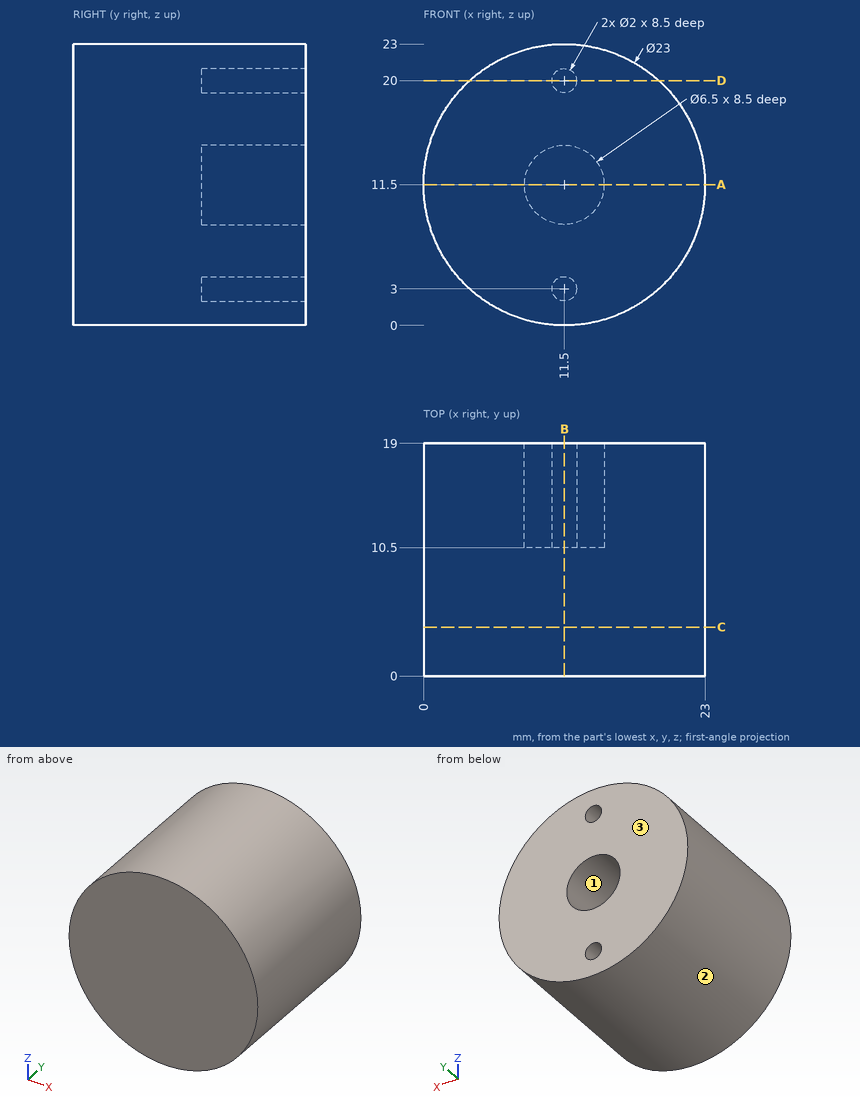
Check sheet for the drawn part. Datum: minimum x, y, z corner. Units: mm. Round coordinates to 2 decimals unless told otherwise and drop trailing zeros. Order: outer loops, then holes, each group sorted by start corner. A loop starts at its lowest first (then second) coordinate and runs counter-clockwise, first axis right, second up. Notation, with made-up numbers: M 12.25,28.5 L 41.25,28.5 A10 ccw 41.25,42.5 Z; hole C 74,17 d5. An arc over 180 degrees is marked long. Write each question's results on one line, items separated by ' | '. Start each with the question number.
1. Go/stop test with flat-tipped pins: P1, Ø0.6, axis at x = 11.5, z = 3, coming from the +Y side; P2, Ø2, axis at x = 13.5, y = 14, coming from the +Z side; P3, Ø1.2, axis at x = 11.5, z = 20, coming from the -Y side; P4, Ø5, axis at y = 5.5, z = 18, coming from the -X side. Record where each tip stops, or that it passes through.
2. Material ranges on L1, parallel to Z at x = 11.5, y = 15; L2, parallel to X at y = 17.5, z = 11.5; L3, parallel to X at y = 17.25, z = 20, recorded low to high. Write a range as from..to.
3. Cross-section at A-A on z = 11.5. Record the boundary of the cut face in (x, y), plus the area to 3 significant figures.
4. Cross-section at B-B on x = 11.5. Record the boundary of the cut face in (y, z).
5. Cross-section at C-C on y = 4. Record the boundary of the cut face in (x, z), plus the area to 3 significant figures.
6. Cross-section at D-D on z = 20. Record the boundary of the cut face in (x, y), plus the area to 3 significant figures.
7. Draft check along Z on the marked faces 1, 2 and 3. Enter one of: pulls with the +Z half, pulls with the -Z half, needs draft (parallel to the pull), parting line crosses it, or undercut.
Resolved:
1) P1: y = 10.5 | P2: z = 22.96 | P3: y = 0 | P4: x = 0.72
2) L1: 0..2, 4..8.25, 14.75..19, 21..23 | L2: 0..8.25, 14.75..23 | L3: 3.75..10.5, 12.5..19.25
3) outline: M 0,0 L 23,0 L 23,19 L 14.75,19 L 14.75,10.5 L 8.25,10.5 L 8.25,19 L 0,19 Z | area: 382 mm2
4) outline: M 0,0 L 19,0 L 19,2 L 10.5,2 L 10.5,4 L 19,4 L 19,8.25 L 10.5,8.25 L 10.5,14.75 L 19,14.75 L 19,19 L 10.5,19 L 10.5,21 L 19,21 L 19,23 L 0,23 Z
5) outline: C 11.5,11.5 d23 | area: 415 mm2
6) outline: M 3.75,0 L 19.25,0 L 19.25,19 L 12.5,19 L 12.5,10.5 L 10.5,10.5 L 10.5,19 L 3.75,19 Z | area: 277 mm2
7) face 1: undercut | face 2: parting line crosses it | face 3: needs draft
